Job drawing, mm, ordinate dimensions from the low corner. One solid piece. Give positions to 0.01 mm unless a question says otherwise; leave off trailing zeros. Loops run counter-clockwise (first coordinate to the right, second up) from the corner with the lowest first, then second, coordinate; pieces in that order, holes last. Notation, with made-up numbers: (46, 44) -> (59, 44) arc R24 ccw to (59, 66) -> close; hole circle Ø8 at (-21.5, -15). An arc over 180 degrees is marked (long way). Answer as a JSON object with one key per item and string values. Group by question number.
Q1. Band-saw the part on A-A, the plane z = 10. Write the cut outline in (x, y).
Q2. Wall check: probe 1 along X at (y, z) = (3.2, 10); probe 2 along X at (y, z) = (0.6, 16.5); probe 3 along Z at (x, y) = (191.5, 3.95). Give the ranges that are in metal, low to high. Write a range as from..to.
Q3. Band-saw the part on C-C, the plane y = 2.3. Write the cut outline in (x, z), plus the area to 3 significant figures.
Q4. Band-saw the part on B-B, the plane x = 191.5. Write the cut outline in (y, z).
Q5. Drop flat-ended pins along their axis: pin 1 (6 mm diameter, centred on x = 191.5, z = 10, fed in from -Y); pin 2 (3 mm diameter, centred on y = 1.5, z = 3, fed in from +X); pin 3 (1.2 mm diameter, centred on x = 199, y = 3.5, fed in from -Z). Give the stop position or say it passes through.
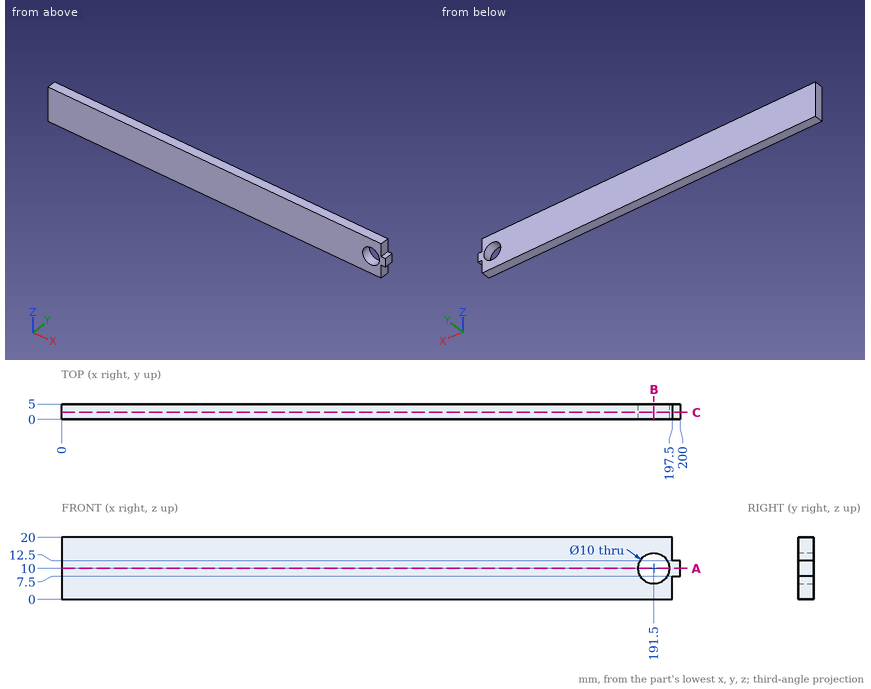
Worked answers:
{
 "1": {"outline": "(0, 0) -> (186.5, 0) -> (186.5, 5) -> (0, 5) -> close; (196.5, 0) -> (200, 0) -> (200, 5) -> (196.5, 5) -> close"},
 "2": {"probe 1": "0..186.5, 196.5..200", "probe 2": "0..197.5", "probe 3": "0..5, 15..20"},
 "3": {"outline": "(0, 0) -> (197.5, 0) -> (197.5, 7.5) -> (200, 7.5) -> (200, 12.5) -> (197.5, 12.5) -> (197.5, 20) -> (0, 20) -> close; hole circle Ø10 at (191.5, 10)", "area": "3,880 mm2"},
 "4": {"outline": "(0, 0) -> (5, 0) -> (5, 5) -> (0, 5) -> close; (0, 15) -> (5, 15) -> (5, 20) -> (0, 20) -> close"},
 "5": {"pin 1": "through", "pin 2": "x = 197.5", "pin 3": "z = 7.5"}
}
